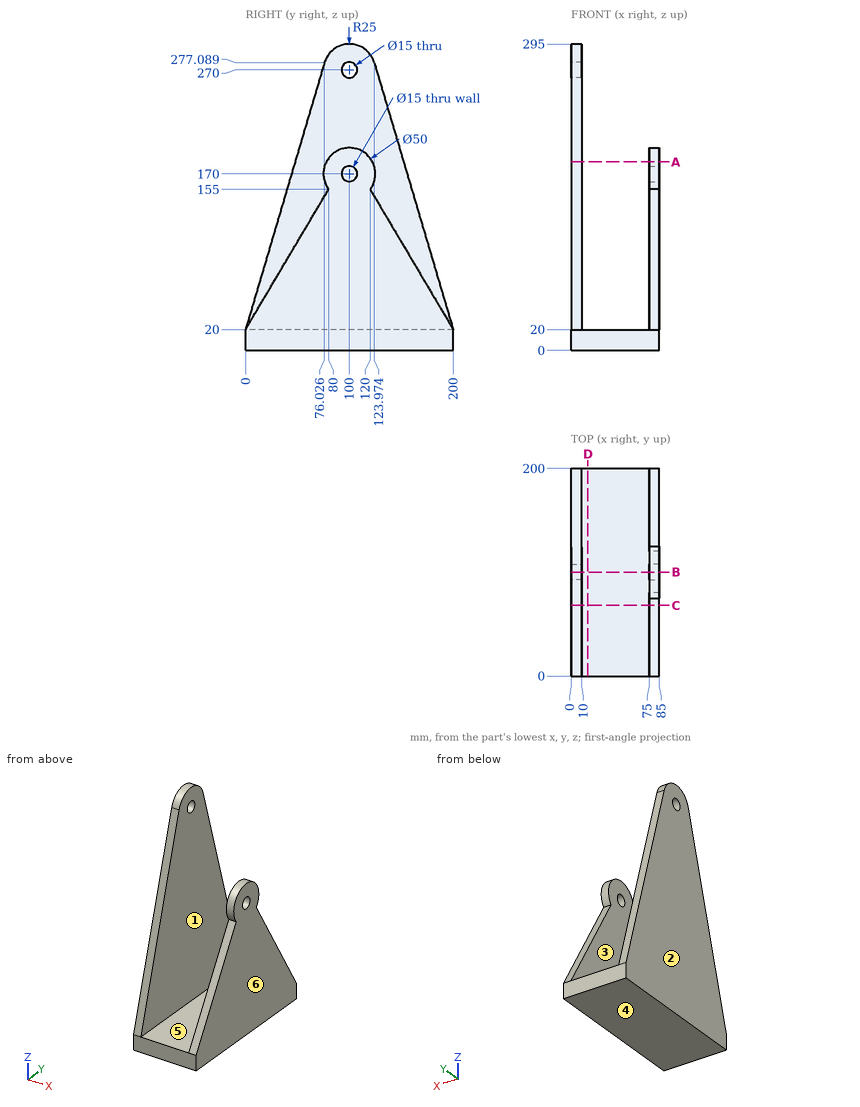
Drawing for the job (mm, zero at the part's lowest x, y, z). A direction names the side the tool comes from. Coordinates: 2 decimals unless noted, no trailing zeros. Order: outer loops, then holes, each group sorted by start corner. A loop starts at its lowest first (then second) coordinate and runs counter-clockwise, first axis right, second up. Notation, with made-up numbers: (-3.75, 57.5) - (11.25, 57.5) arc R29 ccw to (11.25, 91.5) - close; hole circle Ø11 at (-12.75, 34.25). An arc over 180 degrees is marked (long way). Use a Markdown table: item, result. Add a question column.
(1) Drill centre lines: line 1 along X through (y, z) = (71, 101.5); line 2 along Y through (x, z) = (81, 170); line 3 along X through (y, z) = (39.5, 136.5). Where is each one in solid material? Low to high. Write a range as [from, to].
(2) Flat gauge pins, fed straight in: pin 1 (9 mm diameter, centred on y = 100, z = 170, fed in from +X); pin 2 (3 mm diameter, centred on x = 62, y = 124.5, fed in from +Z); pin 3 (12 mm diameter, centred on x = 70, z = 61.5, fed in from -Y). Where does each tip first touch, or does it go through?
(3) Saw through at C-C (y = 68). Give the cut face in (x, z), then the cut area to 3 significant figures.
(4) Which spindle directions (+Z, -Z, +X, -X, +Y, -Y) get a long thin tool onto all of the face, cutting with end or side? Do the marked faces 1 and 2. Say none if no direction does.
(5) Saw through at B-B (y = 100). Give the cut face in (x, z).
(6) Saw through at D-D (x = 16). Give the cut face in (y, z), then the cut area to 3 significant figures.
(7) Pull direction X, two halves, no side cores. Call the marked faces 3, 4, 5 and 6: +X half, -X half, draft (parallel to the pull), parting line (faces both ways), or undercut.
(8) Saw through at A-A (z = 181.5). Give the cut face in (x, y).
Solved:
| question | item | result |
|---|---|---|
| 1 | line 1 | x = [0, 10], [75, 85] |
| 1 | line 2 | y = [75, 92.5], [107.5, 125] |
| 1 | line 3 | x = [0, 10] |
| 2 | pin 1 | stops at x = 10 |
| 2 | pin 2 | stops at z = 20 |
| 2 | pin 3 | stops at y = 22.63 |
| 3 | outline | (0, 0) - (85, 0) - (85, 134.75) - (75, 134.75) - (75, 20) - (10, 20) - (10, 249.95) - (0, 249.95) - close |
| 3 | area | 5,150 mm² |
| 4 | face 1 | +Z, +Y, -Y |
| 4 | face 2 | +Z, -Z, -X, +Y, -Y |
| 5 | outline | (0, 0) - (85, 0) - (85, 162.5) - (75, 162.5) - (75, 20) - (10, 20) - (10, 262.5) - (0, 262.5) - close; (0, 277.5) - (10, 277.5) - (10, 295) - (0, 295) - close; (75, 177.5) - (85, 177.5) - (85, 195) - (75, 195) - close |
| 6 | outline | (0, 0) - (200, 0) - (200, 20) - (0, 20) - close |
| 6 | area | 4,000 mm² |
| 7 | face 3 | undercut |
| 7 | face 4 | draft |
| 7 | face 5 | undercut |
| 7 | face 6 | +X half |
| 8 | outline | (0, 47.76) - (10, 47.76) - (10, 152.24) - (0, 152.24) - close; (75, 77.8) - (85, 77.8) - (85, 122.2) - (75, 122.2) - close |
